Can you work these out from the drawing? Everything is in mm from the part's minimum corner. A direction names the side the tool comes from. Round coordinates to 2 decimals unless told otherwise and drop trailing zeros. Order: outer loops, then holes, each group sorted by start corner. A loop starts at its lowest first (then second) coordinate and runs counter-clockwise, first axis right, second up. Notation, with made-up numbers: (85.25, 67) -> (90.25, 67) arc R33 ccw to (90.25, 104) -> close; hole circle Ø8 at (-3, 20). An arc over 180 degrees is marked (long way). One line per item, written item: value.
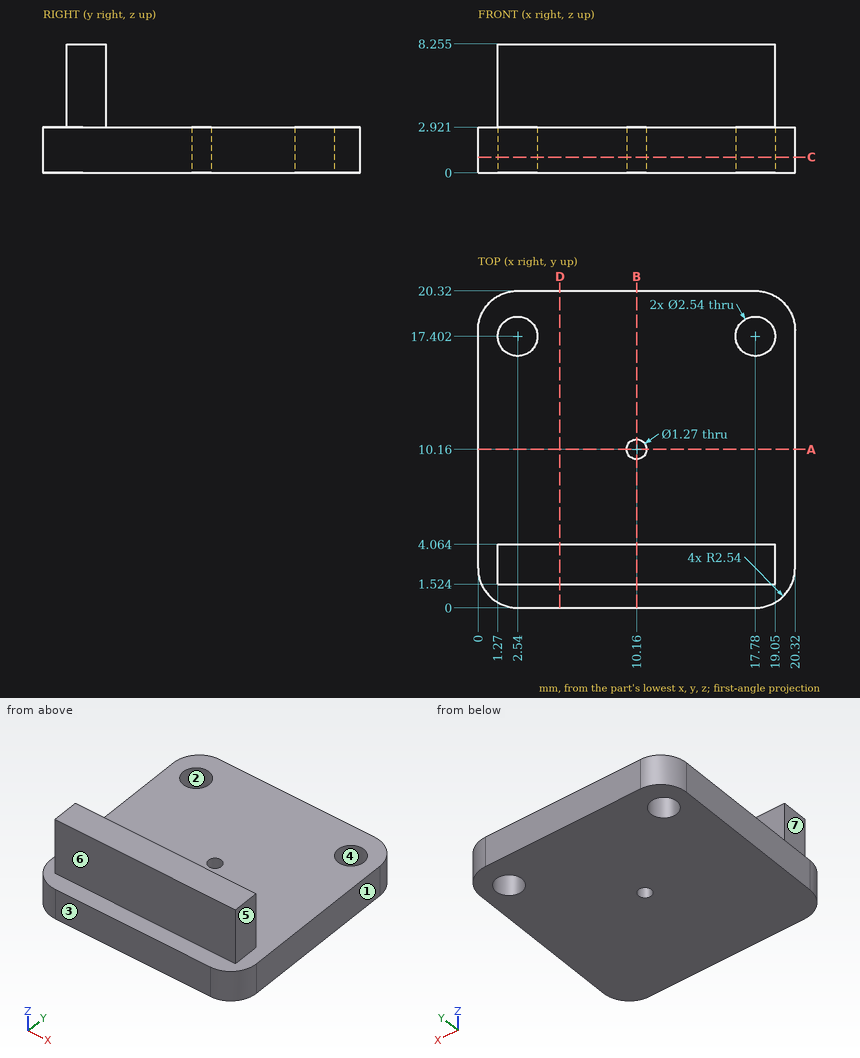
Q1. Which directions (+Z, -Z, +X, -X, +Y, -Y) give clear straight access to the entire face, cutting with the end or side of a thin tool? Please do the marked faces 5, 6 and 7.
Answers:
face 5: +Z, +X, +Y, -Y
face 6: +Z, +X, -X, -Y
face 7: +Z, -X, +Y, -Y
Q2. I want a section at B-B on x = 10.16. Write out the boundary of the cut face in (y, z) (1 decimal).
Answers:
outline: (0, 0) -> (9.5, 0) -> (9.5, 2.9) -> (4.1, 2.9) -> (4.1, 8.3) -> (1.5, 8.3) -> (1.5, 2.9) -> (0, 2.9) -> close; (10.8, 0) -> (20.3, 0) -> (20.3, 2.9) -> (10.8, 2.9) -> close
Q3. For P1, Ø10, axis at x = 14, y = 15, coming from the +Z side; P2, Ø2.5, axis at x = 7, z = 6, coming from the -Y side; P3, Ø2, axis at y = 2.5, z = 5.5, coming from the +X side, each with a flat end and sliding along its axis, tell me the tip position at first contact or that it passes through.
Answers:
P1: z = 2.92
P2: y = 1.52
P3: x = 19.05
Q4. I want a section at A-A on y = 10.16. Write out the boundary of the cut face in (x, z) (1 decimal).
Answers:
outline: (0, 0) -> (9.5, 0) -> (9.5, 2.9) -> (0, 2.9) -> close; (10.8, 0) -> (20.3, 0) -> (20.3, 2.9) -> (10.8, 2.9) -> close
Q5. I want a section at C-C on z = 1. Give the number of separate pieces and of enclosed holes in the cut face, then the cut area to 3 significant figures.
Answers:
separate pieces: 1
enclosed holes: 3
area: 396 mm2
Q6. If we mould it in two halves opening along X, with no side actions, what happens to the marked faces 1, 2, 3 and 4? For each: pulls with the +X half, pulls with the -X half, needs draft (parallel to the pull), parting line crosses it, or undercut.
Answers:
face 1: pulls with the +X half
face 2: undercut
face 3: needs draft
face 4: undercut
Q7. I want a section at D-D on x = 5.25. Write out the boundary of the cut face in (y, z) (1 decimal).
Answers:
outline: (0, 0) -> (20.3, 0) -> (20.3, 2.9) -> (4.1, 2.9) -> (4.1, 8.3) -> (1.5, 8.3) -> (1.5, 2.9) -> (0, 2.9) -> close
Q8. I need wall thicknesses on line 1 along Y through (x, z) = (17.78, 1.2); line 2 along Z through (x, y) = (14, 6.5); line 3 along Y through (x, z) = (11, 6). Which ranges of each line are inside material? Lowest first, please.
Answers:
line 1: 0 to 16.13, 18.67 to 20.32
line 2: 0 to 2.92
line 3: 1.52 to 4.06
